Could you check a few things on this model? Use its own coordinates, in mm. Face numbers are marked on the shaded views. Round coordinates to 2 decimals unless told otherwise and drop trailing zeros. Write each loop counter-clockwise with the first axis right and the second up, starting at its lowest first coordinate (ties: lowest second). Pieces come first, ordered by that corner, then holes. Notation, with made-up numbers: (27.5, 40.5) -> (78.5, 40.5) arc R8 cw to (78.5, 44.5) -> close; hole circle Ø6 at (19, -29.75). An arc over 180 degrees is marked (long way). One line per question, with ' | ' between items. Start each with the question number.
1. Imagine slicing it at B-B, the plane y = 3.35. List the corners of the cut face in (x, z) for me.
2. If I drill on line 1 along Z through (x, y) = (22.5, 2.2); line 2 along X through (y, z) = (1.5, 4); line 3 along Z through (x, y) = (2, 3.35), over which ranges is the centre line in solid material (lowest first)? Write a range as [from, to].
3. Imagine slicing it at C-C, the plane x = 12.5. List the corners of the cut face in (y, z) for me.
4. Thinking about a two-plate mould opening in Z: for the marked faces 1, 2, 3 and 4, which applies, released by +Z, released by -Z, zero draft, split by the parting line, or undercut?
5. Imagine slicing it at D-D, the plane z = 4.75. List the corners of the cut face in (x, y) for me, and give its area (3 significant figures).
6. Imagine slicing it at A-A, the plane z = 7.5. List the corners of the cut face in (x, y) for me, and give its area (3 significant figures).
from build123d import *

# Parameters (mm, degrees)
SKETCH_1_W          = 25
SKETCH_1_H          = 15
EXTRUDE_1_DEPTH     = 4
SKETCH_2_R          = 1.25
SKETCH_2_R_2        = 1.5
CUT_EXTRUDE_1_DEPTH = 4


with BuildPart() as part:
    # 草图1 → 凸台-拉伸1 (new body)
    with BuildSketch(Plane(origin=(0, 0, 0), x_dir=(1, 0, 0), z_dir=(0, 1, 0))):
        with Locations((12.5, -7.5)):
            Rectangle(SKETCH_1_W, SKETCH_1_H)
    extrude(amount=EXTRUDE_1_DEPTH)

    # 草图2 → 切除-拉伸1 (cut)
    with BuildSketch(Plane(origin=(0, 4, 0), x_dir=(1, 0, 0), z_dir=(0, 1, 0))):
        with Locations(Location((2.5, -4, 0), (0, 0, 270))):
            Circle(SKETCH_2_R)
        with Locations(Location((2.5, -11, 0), (0, 0, 270))):
            Circle(SKETCH_2_R)
        with Locations(Location((22.5, -11, 0), (0, 0, 90))):
            Circle(SKETCH_2_R)
        with Locations(Location((22.5, -4, 0), (0, 0, 90))):
            Circle(SKETCH_2_R)
        with Locations(Location((12.5, -7.5, 0), (0, 0, 270))):
            Circle(SKETCH_2_R_2)
    extrude(amount=-CUT_EXTRUDE_1_DEPTH, mode=Mode.SUBTRACT)


solid = part.part
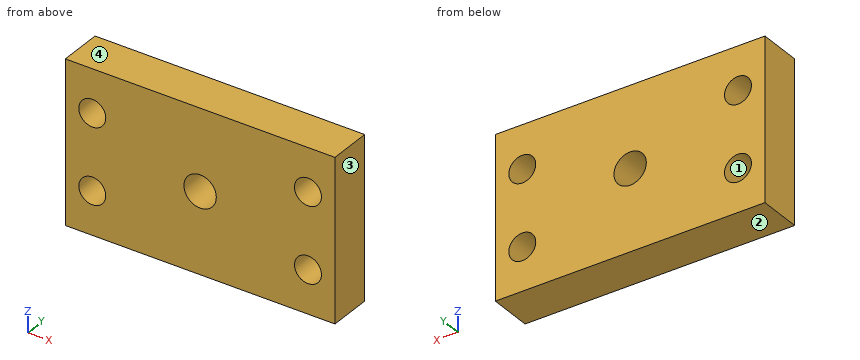
Geometry results:
1) outline: (0, 0) -> (25, 0) -> (25, 15) -> (0, 15) -> close; hole circle Ø2.5 at (2.5, 4); hole circle Ø2.5 at (2.5, 11); hole circle Ø3 at (12.5, 7.5); hole circle Ø2.5 at (22.5, 4); hole circle Ø2.5 at (22.5, 11)
2) line 1: z = [0, 2.75], [5.25, 9.75], [12.25, 15] | line 2: x = [0, 1.25], [3.75, 21.25], [23.75, 25] | line 3: z = [0, 2.85], [5.15, 9.85], [12.15, 15]
3) outline: (0, 0) -> (4, 0) -> (4, 6) -> (0, 6) -> close; (0, 9) -> (4, 9) -> (4, 15) -> (0, 15) -> close
4) face 1: undercut | face 2: released by -Z | face 3: zero draft | face 4: released by +Z
5) outline: (0, 0) -> (1.5, 0) -> (1.5, 4) -> (0, 4) -> close; (3.5, 0) -> (21.5, 0) -> (21.5, 4) -> (3.5, 4) -> close; (23.5, 0) -> (25, 0) -> (25, 4) -> (23.5, 4) -> close | area: 84.0 mm2
6) outline: (0, 0) -> (11, 0) -> (11, 4) -> (0, 4) -> close; (14, 0) -> (25, 0) -> (25, 4) -> (14, 4) -> close | area: 88.0 mm2
